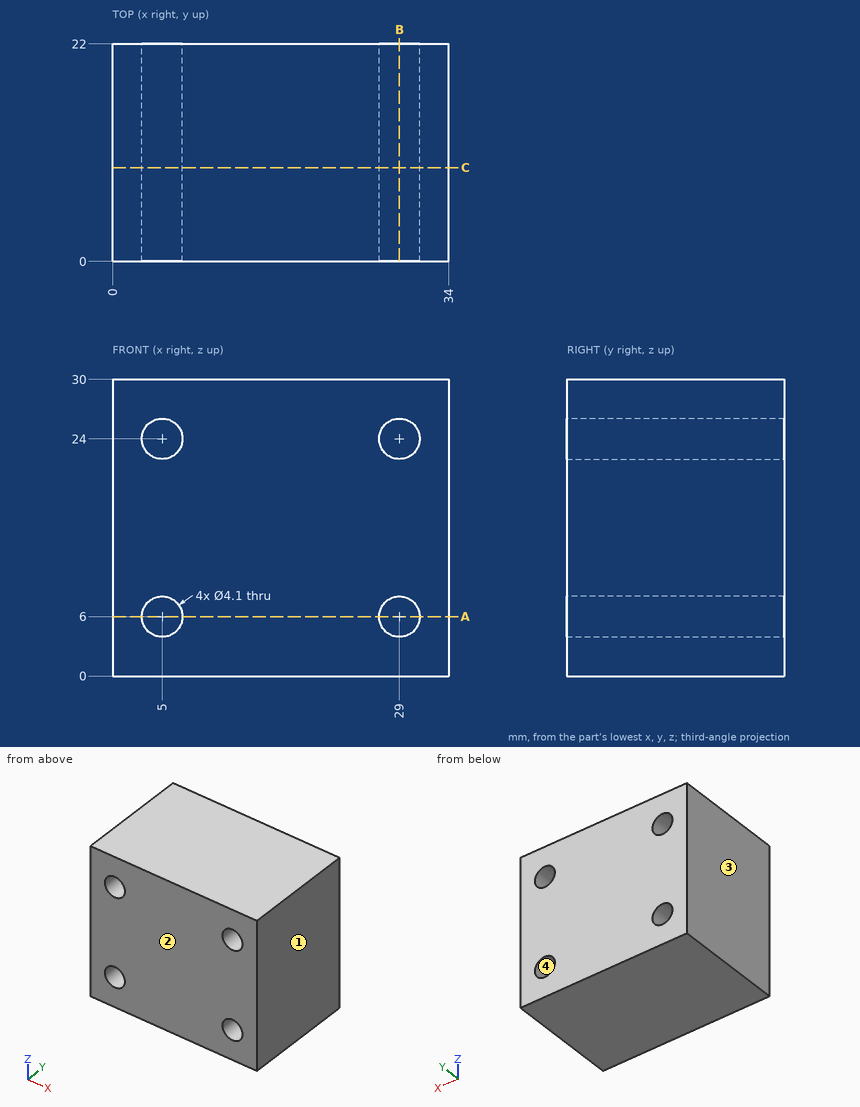
Drawing for the job (mm, zero at the part's lowest x, y, z). Give positions to 0.01 mm unless a question says otherwise; leave off trailing zeros. Loops run counter-clockwise (first coordinate to the right, second up) from the corner with the lowest first, then second, coordinate; pieces in that order, holes last. Notation, with made-up numbers: M 6,11 L 36,11 A21 cw 36,20 Z; hole C 29.25,-33 d11. An arc over 180 degrees is marked long. One line per question, with ' | ' between items. Start each with the question number.
1. Probe L1, parallel to X at y = 15.75, z = 6; L2, parallel to X at y = 9, z = 23.25. List the from-to ranges inside material, lowest first. Write a range as from..to.
2. Flat gauge pin, fed straight in: pin 1 (10 mm diameter, centred on x = 15, y = 13.5, fed in from -Z). Where does the tip first touch, or does it go through?
3. Saw through at A-A on z = 6. Give the cut face in (x, y), plus the area to 3 significant figures.
4. Two-plate mould, pull along X, no slides. Class the marked faces 1, 2, 3 and 4: pulls with the +X half, pulls with the -X half, needs draft (parallel to the pull), parting line crosses it, or undercut.
5. Saw through at C-C on y = 9.5. Give the cut face in (x, z).
6. Saw through at B-B on x = 29. Give the cut face in (y, z).
Result sheet:
1) L1: x = 0..2.95, 7.05..26.95, 31.05..34 | L2: x = 0..3.09, 6.91..27.09, 30.91..34
2) pin 1: stops at z = 0
3) outline: M 0,0 L 2.95,0 L 2.95,22 L 0,22 Z; M 7.05,0 L 26.95,0 L 26.95,22 L 7.05,22 Z; M 31.05,0 L 34,0 L 34,22 L 31.05,22 Z | area: 568 mm^2
4) face 1: pulls with the +X half | face 2: needs draft | face 3: pulls with the -X half | face 4: undercut
5) outline: M 0,0 L 34,0 L 34,30 L 0,30 Z; hole C 5,6 d4.1; hole C 5,24 d4.1; hole C 29,6 d4.1; hole C 29,24 d4.1
6) outline: M 0,0 L 22,0 L 22,3.95 L 0,3.95 Z; M 0,8.05 L 22,8.05 L 22,21.95 L 0,21.95 Z; M 0,26.05 L 22,26.05 L 22,30 L 0,30 Z
